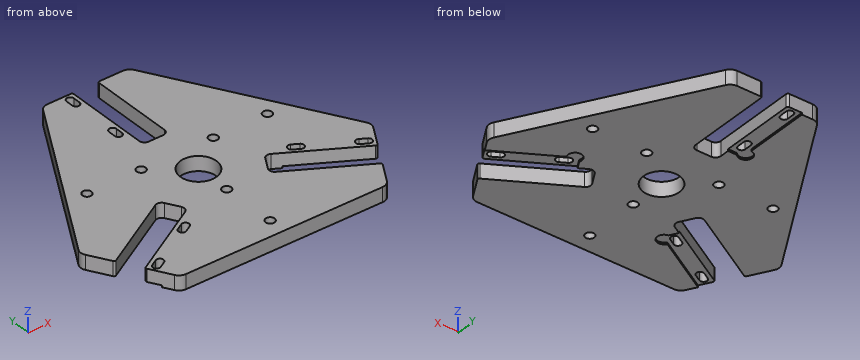
```python
from build123d import *

# Parameters (mm, degrees)
BOSS_EXTRUDE1_DEPTH = 8
SKETCH5_R           = 2.5
SKETCH5_R_2         = 10
CUT_EXTRUDE26_DEPTH = 9
FILLET2_R           = 1
FILLET3_R           = 1
CUT_EXTRUDE27_DEPTH = 1
FILLET4_R           = 1


with BuildPart() as part:
    # Sketch3 → Boss-Extrude1 (new body)
    with BuildSketch(Plane.XY):
        with BuildLine():
            Line((69.282032303, -40), (0, 0))
            Line((0, 0), (-69.282032302, -40))
            Line((-69.282032302, -40), (-58.819418743, -58.121778265))
            ThreePointArc((-58.819418743, -58.121778265), (-56.989291724, -59.951905284), (-54.489291724, -60.621778265))
            Line((-54.489291724, -60.621778265), (54.489291724, -60.621778265))
            ThreePointArc((54.489291724, -60.621778265), (56.989291724, -59.951905284), (58.819418743, -58.121778265))
            Line((58.819418743, -58.121778265), (69.282032303, -40))
        make_face()
        with BuildLine():
            Line((0, 80), (0, 0))
            Line((0, 0), (69.282032303, -40))
            Line((69.282032303, -40), (79.744645862, -21.878221735))
            ThreePointArc((79.744645862, -21.878221735), (80.414518843, -19.378221735), (79.744645862, -16.878221735))
            Line((79.744645862, -16.878221735), (25.255354138, 77.5))
            ThreePointArc((25.255354138, 77.5), (23.425227119, 79.330127019), (20.925227119, 80))
            Line((20.925227119, 80), (0, 80))
        make_face()
        with BuildLine():
            Line((-69.282032302, -40), (0, 0))
            Line((0, 0), (0, 80))
            Line((0, 80), (-20.925227119, 80))
            ThreePointArc((-20.925227119, 80), (-23.425227119, 79.330127019), (-25.255354138, 77.5))
            Line((-25.255354138, 77.5), (-79.744645862, -16.878221735))
            ThreePointArc((-79.744645862, -16.878221735), (-80.414518843, -19.378221735), (-79.744645862, -21.878221735))
            Line((-79.744645862, -21.878221735), (-69.282032302, -40))
        make_face()
    extrude(amount=BOSS_EXTRUDE1_DEPTH)

    # Sketch5 → Cut-Extrude26 (cut, through all)
    with BuildSketch(Plane.XY.offset(8)):
        with BuildLine():
            Line((6.99085892, 80), (-7.00914108, 80))
            Line((-7.00914108, 80), (-7.00914108, 32.993673427))
            ThreePointArc((-7.00914108, 32.993673427), (-6.130461423, 30.872353083), (-4.00914108, 29.993673427))
            Line((-4.00914108, 29.993673427), (3.99085892, 29.993673427))
            ThreePointArc((3.99085892, 29.993673427), (6.112179264, 30.872353083), (6.99085892, 32.993673427))
            Line((6.99085892, 32.993673427), (6.99085892, 80))
        make_face()
        with BuildLine():
            Line((-13.00914108, 76.493673427), (-13.00914108, 72.493673427))
            ThreePointArc((-13.00914108, 72.493673427), (-11.00914108, 70.493673427), (-9.00914108, 72.493673427))
            Line((-9.00914108, 72.493673427), (-9.00914108, 76.493673427))
            ThreePointArc((-9.00914108, 76.493673427), (-11.00914108, 78.493673427), (-13.00914108, 76.493673427))
        make_face()
        with BuildLine():
            Line((-13.00914108, 46.493673427), (-13.00914108, 42.493673427))
            ThreePointArc((-13.00914108, 42.493673427), (-11.00914108, 40.493673427), (-9.00914108, 42.493673427))
            Line((-9.00914108, 42.493673427), (-9.00914108, 46.493673427))
            ThreePointArc((-9.00914108, 46.493673427), (-11.00914108, 48.493673427), (-13.00914108, 46.493673427))
        make_face()
        with Locations((49.99085892, 14.993673427)):
            Circle(SKETCH5_R)
        with Locations((19.99085892, 14.993673427)):
            Circle(SKETCH5_R)
        with Locations((-20.00914108, 14.993673427)):
            Circle(SKETCH5_R)
        with Locations((-50.00914108, 14.993673427)):
            Circle(SKETCH5_R)
        with Locations((-0.00914108, -0.006326573)):
            Circle(SKETCH5_R_2)
        with BuildLine():
            Line((-32.087979405, -10.444148747), (-72.781578086, -33.9386089))
            Line((-72.781578086, -33.9386089), (-65.781578086, -46.062964553))
            Line((-65.781578086, -46.062964553), (-25.087979405, -22.5685044))
            ThreePointArc((-25.087979405, -22.5685044), (-23.690201926, -20.746885324), (-23.989903193, -18.470428188))
            Line((-23.989903193, -18.470428188), (-27.989903193, -11.542224958))
            ThreePointArc((-27.989903193, -11.542224958), (-29.811522269, -10.144447479), (-32.087979405, -10.444148747))
        make_face()
        with BuildLine():
            Line((-33.779322356, -34.514656822), (-30.315220741, -32.514656822))
            ThreePointArc((-30.315220741, -32.514656822), (-29.583169933, -29.782606015), (-32.315220741, -29.050555207))
            Line((-32.315220741, -29.050555207), (-35.779322356, -31.050555207))
            ThreePointArc((-35.779322356, -31.050555207), (-36.511373163, -33.782606015), (-33.779322356, -34.514656822))
        make_face()
        with BuildLine():
            Line((-59.760084469, -49.514656822), (-56.295982854, -47.514656822))
            ThreePointArc((-56.295982854, -47.514656822), (-55.563932046, -44.782606015), (-58.295982854, -44.050555207))
            Line((-58.295982854, -44.050555207), (-61.760084469, -46.050555207))
            ThreePointArc((-61.760084469, -46.050555207), (-62.492135277, -48.782606015), (-59.760084469, -49.514656822))
        make_face()
        with Locations((-0.00914108, -50.628104838)):
            Circle(SKETCH5_R)
        with Locations((-0.00914108, -20.006326573)):
            Circle(SKETCH5_R)
        with BuildLine():
            Line((65.777007546, -46.07088096), (72.777007546, -33.946525307))
            Line((72.777007546, -33.946525307), (32.069697245, -10.444148747))
            ThreePointArc((32.069697245, -10.444148747), (29.793240109, -10.144447479), (27.971621033, -11.542224958))
            Line((27.971621033, -11.542224958), (23.971621033, -18.470428188))
            ThreePointArc((23.971621033, -18.470428188), (23.671919766, -20.746885324), (25.069697245, -22.5685044))
            Line((25.069697245, -22.5685044), (65.777007546, -46.07088096))
        make_face()
        with BuildLine():
            Line((41.296938581, -13.462097939), (44.761040196, -15.462097939))
            ThreePointArc((44.761040196, -15.462097939), (47.493091003, -14.730047132), (46.761040196, -11.997996324))
            Line((46.761040196, -11.997996324), (43.296938581, -9.997996324))
            ThreePointArc((43.296938581, -9.997996324), (40.564887773, -10.730047132), (41.296938581, -13.462097939))
        make_face()
        with BuildLine():
            Line((67.277700694, -28.462097939), (70.741802309, -30.462097939))
            ThreePointArc((70.741802309, -30.462097939), (73.473853117, -29.730047132), (72.741802309, -26.997996324))
            Line((72.741802309, -26.997996324), (69.277700694, -24.997996324))
            ThreePointArc((69.277700694, -24.997996324), (66.545649887, -25.730047132), (67.277700694, -28.462097939))
        make_face()
    extrude(amount=-CUT_EXTRUDE26_DEPTH, mode=Mode.SUBTRACT)

    # Fillet2
    fillet2_edges = [part.edges().sort_by_distance(p)[0] for p in [
        (72.777007546, -33.946525307, 4),
    ]]
    fillet(fillet2_edges, radius=FILLET2_R)

    # Fillet3
    fillet3_edges = [part.edges().sort_by_distance(p)[0] for p in [
        (-65.781578086, -46.062964553, 4),
        (-72.781578086, -33.9386089, 4),
        (65.777007546, -46.07088096, 4),
        (-7.00914108, 80, 4),
        (6.99085892, 80, 4),
    ]]
    fillet(fillet3_edges, radius=FILLET3_R)

    # Sketch7 → Cut-Extrude27 (cut)
    with BuildSketch(Plane(origin=(0, 0, 0), x_dir=(-1, 0, 0), z_dir=(0, 0, -1))):
        with BuildLine():
            Line((61.781578086, -52.991167783), (30.60466355, -34.991167783))
            ThreePointArc((30.60466355, -34.991167783), (24.227648547, -35.182379801), (26.908511127, -29.393091572))
            Line((26.908511127, -29.393091572), (29.408511127, -25.062964553))
            Line((29.408511127, -25.062964553), (65.781578086, -46.062964553))
            Line((65.781578086, -46.062964553), (61.781578086, -52.991167783))
        make_face()
        with BuildLine():
            Line((-76.777007546, -27.018322077), (-45.60009301, -9.018322077))
            ThreePointArc((-45.60009301, -9.018322077), (-42.577179974, -3.400059076), (-38.903940587, -8.616398288))
            Line((-38.903940587, -8.616398288), (-36.403940587, -12.946525307))
            Line((-36.403940587, -12.946525307), (-72.777007546, -33.946525307))
            Line((-72.777007546, -33.946525307), (-76.777007546, -27.018322077))
        make_face()
        with BuildLine():
            Line((15.00914108, 80), (15.00914108, 44))
            ThreePointArc((15.00914108, 44), (18.363243046, 38.572949017), (12.00914108, 38))
            Line((12.00914108, 38), (7.00914108, 38))
            Line((7.00914108, 38), (7.00914108, 80))
            Line((7.00914108, 80), (15.00914108, 80))
        make_face()
    extrude(amount=-CUT_EXTRUDE27_DEPTH, mode=Mode.SUBTRACT)

    # Fillet4
    fillet4_edges = [part.edges().sort_by_distance(p)[0] for p in [
        (45.60009301, -9.018322077, 0.5),
        (-30.60466355, -34.991167783, 0.5),
        (-15.00914108, 44, 0.5),
    ]]
    fillet(fillet4_edges, radius=FILLET4_R)


solid = part.part
```
Geometry check sheet. Reference: the model listing, model coordinates, mm. Coordinates: 2 decimals unless noted, no trailing zeros. Write each loop counter-clockwise with the first axis right and the second up, starting at its lowest first coordinate (ties: lowest second). Pieces come first, ordered by that corner, then holes. Notation, with made-up numbers: M 8,70.25 L 45,70.25 A11 ccw 45,75.25 Z; hole C 8,61 d1. An arc over 180 degrees is marked long. Answer as a JSON object with one key per item and string values.
1. Section check C-C, the plane z = 4. Give the number of separate pieces and of enclosed holes in the cut face, plus the area to 3 significant figures.
Answers below:
{"separate pieces": "1", "enclosed holes": "13", "area": "13,400 mm²"}
2. Go/stop test with flat-tipped pins: pin 1 Ø0.8 at (x, z) = (-10.5, 0.5) entering from +Y; pin 2 Ø1.2 at (y, z) = (45.5, 6) entering from +X; pin 3 Ø4 at (x, z) = (-0.5, 2.5) entering from +Y; pin 4 Ø4 at (x, y) = (-50.01, 14.99) entering from -Z. Record where each tip stops, or that it passes through.
Answers below:
{"pin 1": "stops at y = 38", "pin 2": "stops at x = 44.08", "pin 3": "stops at y = 29.99", "pin 4": "passes through"}
3. Section check B-B, the plane x = 50. Enter the section's corners in (y, z), plus the area to 3 significant figures.
Answers below:
{"outline": "M -60.62,0 L -36.96,0 L -36.96,8 L -60.62,8 Z; M -20.8,1 L -11.56,1 L -11.56,0 L 12.49,0 L 12.49,8 L -20.8,8 Z; M 17.49,0 L 34.64,0 L 34.64,8 L 17.49,8 Z", "area": "584 mm²"}
4. Section check A-A, the plane y = 57.5. Enter the section's corners in (x, z).
Answers below:
{"outline": "M -36.8,0 L -15.01,0 L -15.01,1 L -7.01,1 L -7.01,8 L -36.8,8 Z; M 6.99,0 L 36.8,0 L 36.8,8 L 6.99,8 Z"}
5. Scan lines: L1, parallel to Y at x = -11, z = 2.5; L2, parallel to X at y = -14, z = 4.75; L3, parallel to Y at x = -45, z = 1.75. Record each from-to range of solid material in increasing order.
Answers below:
{"L1": "y = -60.62 to 40.49, 48.49 to 70.49, 78.49 to 80", "L2": "x = -78.08 to -38.25, -26.57 to 26.55, 38.23 to 42.23, 47.74 to 78.08", "L3": "y = -60.62 to -34.06, -17.9 to 43.3"}
